Study the drawing (mm; zero at the part's minimum x, y, z) and answer. Coordinates: 2 decimals unless noted, no trailing zeros. Loops run counter-clockwise (first coordinate to the right, second up) from the corner with the lowest first, then second, coordinate; pieces in that order, holes last.
Q1. Section C-C (z = 3.5) is taken. Give the vertices of the cut face in (x, y) (1 decimal).
Q2. The mould has two halves that part along Z. Classify the marked faces 1, 2 and 3: pulls with the +Z half, pulls with the -Z half, needs draft (parallel to the pull), parting line crosses it, or undercut.
Q3. Section B-B (x = 45) is taken. Give the vertices of the cut face in (y, z).
Q4. Section A-A (z = 15) is taken. Give the vertices of the cut face in (x, y), then the cut area to 3 significant figures.
Q5. Section D-D (y = 8) is taken. Count the separate pieces of the cut face and the enclosed holes in it, then the cut area to 3 significant figures.
Q6. Straight lines are drawn through the part: line 1 (X direction, y = 7, z = 5); line 2 (Z direction, x = 45, y = 8); line 3 (X direction, y = 6.5, z = 3.25) (1 decimal). For each, find the intervals that lie inside material, in ascending order.
Q7. A flat-ended cylindrical pin translates along its axis: P1, Ø4, axis at x = 45, z = 5, coming from the +Y side. Find the tip coordinate at first contact, or state that the pin passes through.
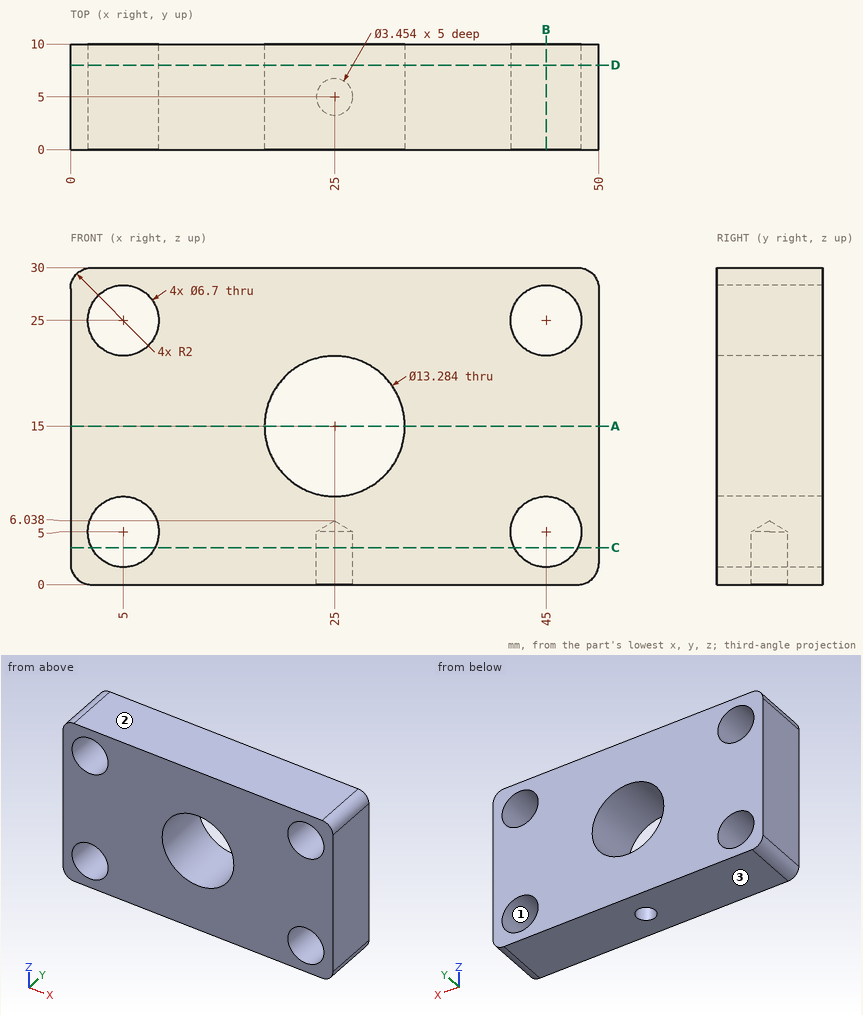
Numbers:
1. outline: (0, 0) - (2, 0) - (2, 10) - (0, 10) - close; (8, 0) - (42, 0) - (42, 10) - (8, 10) - close; (48, 0) - (50, 0) - (50, 10) - (48, 10) - close; hole circle Ø3.5 at (25, 5)
2. face 1: undercut
2. face 2: pulls with the +Z half
2. face 3: pulls with the -Z half
3. outline: (0, 0) - (10, 0) - (10, 1.65) - (0, 1.65) - close; (0, 8.35) - (10, 8.35) - (10, 21.65) - (0, 21.65) - close; (0, 28.35) - (10, 28.35) - (10, 30) - (0, 30) - close
4. outline: (0, 0) - (18.36, 0) - (18.36, 10) - (0, 10) - close; (31.64, 0) - (50, 0) - (50, 10) - (31.64, 10) - close
4. area: 367 mm2
5. separate pieces: 1
5. enclosed holes: 5
5. area: 1,220 mm2
6. line 1: x = 0 to 1.65, 8.35 to 41.65, 48.35 to 50
6. line 2: z = 0 to 1.65, 8.35 to 21.65, 28.35 to 30
6. line 3: x = 0 to 2.1, 7.9 to 24.1, 25.9 to 42.1, 47.9 to 50
7. P1: passes through
